Design review of the part built by this model. Coordinates are the model's own, in mm. Round coordinates to 2 decimals unless told otherwise and drop trailing zeros. Return JSON: item names as keys, results as strings. Group by question number.
(1) The part is to be moulded in two halves that separate along X. For faces 1 (the flat face through (-5, 395, 9)), 2 (the cylindrical face through (-161.49, -139.49, 16.02)), 3 (the flat face through (50, 155, 14.5)), say which applies: pulls with the +X half, pulls with the -X half, needs draft (parallel to the pull), parting line crosses it, or undercut.
(2) Clearance check with a flat-ended pin moving along its axis: pin 1 (18.5 mm diameter, centred on x = -50, y = -240, fed in from +Z). State where the tip first meets the part, or that it passes through.
(3) Wall thickness on L1, parallel to Z at x = -154, y = 250.5: over which ranges is the line inside the solid? List them lowest first. Write a range as [from, to].
from build123d import *

# Parameters (mm, degrees)
F0_W           = 730
F0_H           = 790
F1_DEPTH       = 17.5
F3_D           = 9
F3_CBORE_D     = 23
F3_CBORE_DEPTH = 3


# Not quite as in the source:
# - a feature names something its author has since deleted; it is built from what else it names


with BuildPart() as f1:
    # F0 (on Top) → F1 (new body)
    with BuildSketch(Plane.XY):
        Rectangle(F0_W, F0_H)
    extrude(amount=F1_DEPTH)

    # F3 (through all)
    with Locations(Plane.XY.offset(17.5)):
        with Locations((-250, 260), (-150, 260), (-50, 260), (50, 260), (150, 260), (-150, 160), (-250, 60), (-250, 160), (150, 60), (-150, -140), (-150, -40), (150, -140), (50, -140), (-150, 60), (-50, 60), (-50, -140), (-250, -140), (50, 160), (50, -40), (-250, -40), (150, 160), (150, -40), (-50, 160), (-50, -40), (50, 60), (250, 260), (250, 160), (250, 60), (250, -40), (250, -140), (250, -240), (150, -240), (50, -240), (-50, -240), (-150, -240), (-250, -240)):
            CounterBoreHole(F3_D / 2, F3_CBORE_D / 2, F3_CBORE_DEPTH)


solid = f1.part
Solutions:
{
 "1": {"face 1": "needs draft", "face 2": "undercut", "face 3": "undercut"},
 "2": {"pin 1": "z = 14.5"},
 "3": {"L1": "[0, 14.5]"}
}
